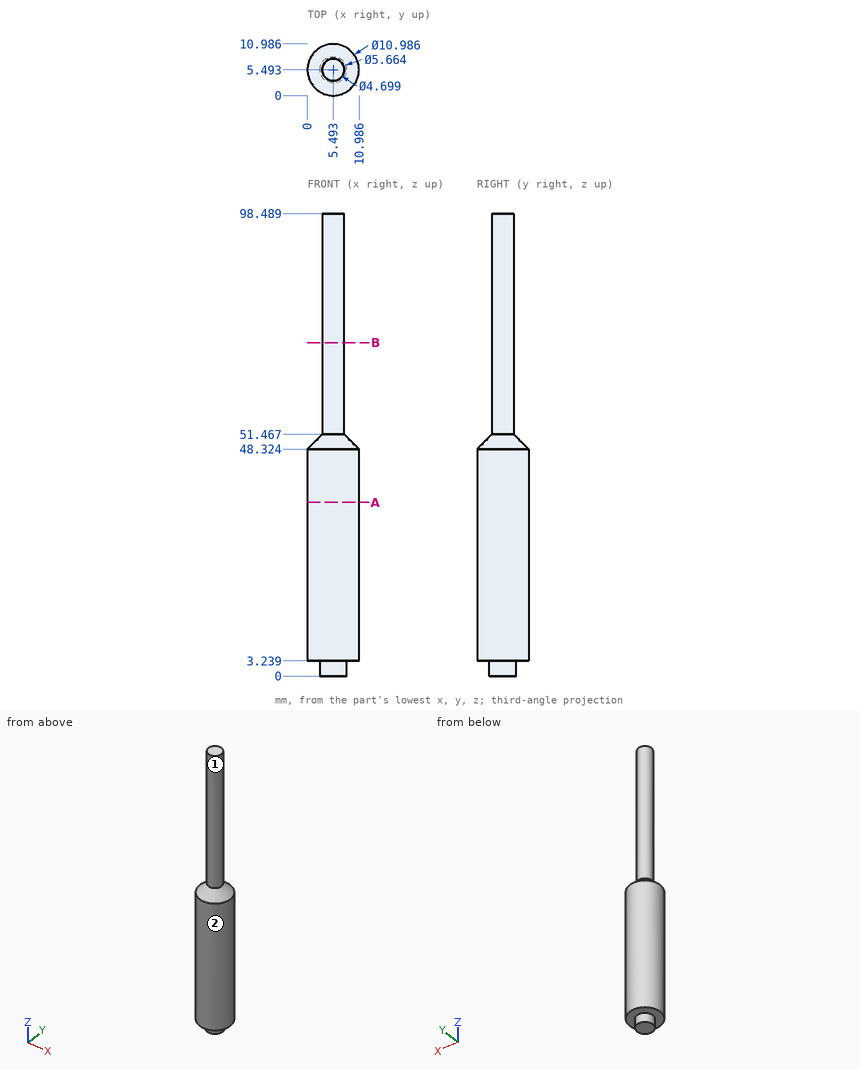
Print and shaded views of the part. All mm, measured from the part's lowest x, y and z. A direction names the side the tool comes from. Coordinates: 2 decimals unless noted, no trailing zeros. Order: outer loops, then holes, each group sorted by start corner. A loop starts at its lowest first (then second) coordinate and runs counter-clockwise, first axis right, second up. Notation, with made-up numbers: (16, 17.5) - (26, 17.5) arc R8 cw to (26, 31.5) - close; hole circle Ø4 at (-24.75, 54). An arc over 180 degrees is marked (long way). Return JSON: item names as keys, results as strings. Group by question number.
Item 1: Pin check, flat tips, straight feed: pin 1 (1.5 mm diameter, centred on x = 6.5, z = 54, fed in from +Y); pin 2 (1 mm diameter, centred on x = 9.5, y = 8.5, fed in from +Z) (1 decimal); pin 3 (6 mm diameter, centred on y = 6, z = 62, fed in from -X). Stop position of each tip, or through.
Item 2: Cut at B-B (z = 71). List the corners of the cut face in (x, y).
Item 3: Cut at A-A (z = 37). List the corners of the cut face in (x, y) (1 decimal).
Item 4: Drill centre lines: probe 1 along Y at (x, z) = (5.75, 30) (1 decimal); probe 2 along Y at (x, z) = (5.5, 87). Where is each one in solid material? Low to high. Write a range as from..to.
Item 5: Which spindle directions (+Z, -Z, +X, -X, +Y, -Y) get a long thin tool onto all of the face, cutting with end or side? Do the marked faces 1 and 2. Say none if no direction does.
Check values:
{
 "1": {"pin 1": "stops at y = 7.83", "pin 2": "stops at z = 49.3", "pin 3": "stops at x = 3.14"},
 "2": {"outline": "circle Ø4.7 at (5.49, 5.49)"},
 "3": {"outline": "circle Ø11 at (5.5, 5.5)"},
 "4": {"probe 1": "y = 0..11", "probe 2": "y = 3.14..7.84"},
 "5": {"face 1": "+Z", "face 2": "+Z, -Z"}
}
